from build123d import *

# Parameters (mm, degrees)
SKETCH_1_R                = 7
EXTRUDE_1_DEPTH           = 54
SKETCH_2_R                = 5
EXTRUDE_2_DEPTH           = 7
CHAMFER_1_SIZE            = 1
SKETCH_3_R                = 10
EXTRUDE_3_DEPTH           = 2
SKETCH_4_R                = 6
EXTRUDE_4_DEPTH           = 25
SKETCH_7_R                = 10
EXTRUDE_5_DEPTH           = 4.3
SKETCH_9_R                = 10
SKETCH_9_R_2              = 6
CUT_EXTRUDE_3_DEPTH       = 1.3
SKETCH_11_R               = 27
SKETCH_11_R_2             = 10
EXTRUDE_6_DEPTH           = 5
SKETCH_12_R               = 9.5
SKETCH_12_R_2             = 6
EXTRUDE_7_DEPTH           = 30
SKETCH_14_R               = 2.5
CUT_EXTRUDE_4_DEPTH       = 10
CUT_EXTRUDE_5_DEPTH       = 30
CHAMFER_2_SIZE            = 1
HOLE_WIZARD_M3_1_D        = 2.5
HOLE_WIZARD_M3_1_DEPTH    = 18.5
HOLE_WIZARD_M3_1_TIP      = 0.751075774
SKETCH_22_W               = 38.47112098
SKETCH_22_H               = 24.703275639
CUT_EXTRUDE_10_DEPTH      = 28
CUT_EXTRUDE_10_DEPTH_BACK = 28
SKETCH_24_R               = 9.5
EXTRUDE_9_DEPTH           = 10.3
SKETCH_25_R               = 7.5
EXTRUDE_10_DEPTH          = 17
SKETCH_26_W               = 19.870375241
SKETCH_26_H               = 17.333591793
CUT_EXTRUDE_11_DEPTH      = 28
CUT_EXTRUDE_11_DEPTH_BACK = 28
SKETCH_27_R               = 9.5
EXTRUDE_11_DEPTH          = 7.7
SKETCH_29_R               = 7.5
EXTRUDE_12_DEPTH          = 10
CUT_EXTRUDE_12_REACH      = 82
HOLE_WIZARD_M4_1_D        = 3.3
CHAMFER_4_SIZE            = 1
SKETCH_33_R               = 9.5
SKETCH_33_R_2             = 8.5
CUT_EXTRUDE_13_DEPTH      = 10
SKETCH_34_R               = 9.5
SKETCH_34_R_2             = 8.5
CUT_EXTRUDE_14_DEPTH      = 7.7
SKETCH_35_W               = 0.25
SKETCH_35_H               = 0.5
SKETCH_36_W               = 0.25
SKETCH_36_H               = 0.5


with BuildPart() as part:
    # 草图1 → 凸台-拉伸1 (new body)
    with BuildSketch(Plane.XY):
        Circle(SKETCH_1_R)
    extrude(amount=EXTRUDE_1_DEPTH)

    # 草图2 → 凸台-拉伸2 (add)
    with BuildSketch(Plane.XY.offset(54)):
        Circle(SKETCH_2_R)
    extrude(amount=EXTRUDE_2_DEPTH)

    # 倒角1
    chamfer_1_edges = [part.edges().sort_by_distance(p)[0] for p in [
        (-5, 0, 61),
    ]]
    chamfer(chamfer_1_edges, length=CHAMFER_1_SIZE)

    # 草图3 → 凸台-拉伸3 (add)
    with BuildSketch(Plane.XY.offset(42)):
        Circle(SKETCH_3_R)
    extrude(amount=-EXTRUDE_3_DEPTH)

    # 草图4 → 凸台-拉伸4 (add)
    with BuildSketch(Plane(origin=(0, 0, 0), x_dir=(-1, 0, 0), z_dir=(0, 0, -1))):
        Circle(SKETCH_4_R)
    extrude(amount=EXTRUDE_4_DEPTH)

    # 草图7 → 凸台-拉伸5 (add)
    with BuildSketch(Plane.XY.offset(42)):
        Circle(SKETCH_7_R)
    extrude(amount=EXTRUDE_5_DEPTH)

    # 草图9 → 切除-拉伸3 (cut)
    with BuildSketch(Plane(origin=(0, 0, 40), x_dir=(-1, 0, 0), z_dir=(0, 0, -1))):
        Circle(SKETCH_9_R)
        Circle(SKETCH_9_R_2, mode=Mode.SUBTRACT)
    extrude(amount=-CUT_EXTRUDE_3_DEPTH, mode=Mode.SUBTRACT)

    # 草图11 → 凸台-拉伸6 (add)
    with BuildSketch(Plane.XY.offset(46.3)):
        Circle(SKETCH_11_R)
        Circle(SKETCH_11_R_2, mode=Mode.SUBTRACT)
    extrude(amount=-EXTRUDE_6_DEPTH)

    # 草图12 → 凸台-拉伸7 (add)
    with BuildSketch(Plane(origin=(0, 0, 41.3), x_dir=(-1, 0, 0), z_dir=(0, 0, -1))):
        Circle(SKETCH_12_R)
        Circle(SKETCH_12_R_2, mode=Mode.SUBTRACT)
    extrude(amount=EXTRUDE_7_DEPTH)

    # 草图14 → 切除-拉伸4 (cut)
    with BuildSketch(Plane.XY.offset(46.3)):
        with Locations((22.5, 0)):
            Circle(SKETCH_14_R)
        with Locations((11.25, -19.485571585)):
            Circle(SKETCH_14_R)
        with Locations((-11.25, -19.485571585)):
            Circle(SKETCH_14_R)
        with Locations((-22.5, 0)):
            Circle(SKETCH_14_R)
        with Locations((-11.25, 19.485571585)):
            Circle(SKETCH_14_R)
        with Locations((11.25, 19.485571585)):
            Circle(SKETCH_14_R)
    extrude(amount=-CUT_EXTRUDE_4_DEPTH, mode=Mode.SUBTRACT)

    # 草图13 → 切除-拉伸5 (cut)
    with BuildSketch(Plane(origin=(0, 0, -25), x_dir=(-1, 0, 0), z_dir=(0, 0, -1))):
        with BuildLine():
            Line((2.15, 2.092247595), (2.15, -2.092247595))
            ThreePointArc((2.15, -2.092247595), (0, -3), (-2.15, -2.092247595))
            Line((-2.15, -2.092247595), (-2.15, 2.092247595))
            ThreePointArc((-2.15, 2.092247595), (0, 3), (2.15, 2.092247595))
        make_face()
    extrude(amount=-CUT_EXTRUDE_5_DEPTH, mode=Mode.SUBTRACT)

    # 倒角2
    chamfer_2_edges = [part.edges().sort_by_distance(p)[0] for p in [
        (6, 0, -25),
    ]]
    chamfer(chamfer_2_edges, length=CHAMFER_2_SIZE)

    # M3 螺纹孔1
    with Locations(Plane(origin=(7.85, 0, -17), x_dir=(0, 0, 1), z_dir=(1, 0, 0))):
        with Locations((0, 0)):
            Hole(HOLE_WIZARD_M3_1_D / 2, depth=HOLE_WIZARD_M3_1_DEPTH)
            with Locations((0, 0, -(HOLE_WIZARD_M3_1_DEPTH + HOLE_WIZARD_M3_1_TIP / 2))):  # 118° drill point
                Cone(0, HOLE_WIZARD_M3_1_D / 2, HOLE_WIZARD_M3_1_TIP, mode=Mode.SUBTRACT)

    # 草图22 → 切除-拉伸10 (cut, two sides)
    with BuildSketch(Plane(origin=(0, 0, 0), x_dir=(0, 0, -1), z_dir=(1, 0, 0))) as cut_extrude_10_sk:
        with Locations((7.93556049, 2.744045787)):
            Rectangle(SKETCH_22_W, SKETCH_22_H)
    extrude(amount=CUT_EXTRUDE_10_DEPTH, mode=Mode.SUBTRACT)
    extrude(cut_extrude_10_sk.sketch, amount=-CUT_EXTRUDE_10_DEPTH_BACK, mode=Mode.SUBTRACT)

    # 草图24 → 凸台-拉伸9 (add)
    with BuildSketch(Plane(origin=(0, 0, 11.3), x_dir=(-1, 0, 0), z_dir=(0, 0, -1))):
        Circle(SKETCH_24_R)
    extrude(amount=EXTRUDE_9_DEPTH)

    # 草图25 → 凸台-拉伸10 (add)
    with BuildSketch(Plane(origin=(0, 0, 1), x_dir=(-1, 0, 0), z_dir=(0, 0, -1))):
        Circle(SKETCH_25_R)
    extrude(amount=EXTRUDE_10_DEPTH)

    # 草图26 → 切除-拉伸11 (cut, two sides)
    with BuildSketch(Plane(origin=(0, 0, 0), x_dir=(0, 0, -1), z_dir=(1, 0, 0))) as cut_extrude_11_sk:
        with Locations((-56.23518762, 1.256529054)):
            Rectangle(SKETCH_26_W, SKETCH_26_H)
    extrude(amount=CUT_EXTRUDE_11_DEPTH, mode=Mode.SUBTRACT)
    extrude(cut_extrude_11_sk.sketch, amount=-CUT_EXTRUDE_11_DEPTH_BACK, mode=Mode.SUBTRACT)

    # 草图27 → 凸台-拉伸11 (add)
    with BuildSketch(Plane.XY.offset(46.3)):
        Circle(SKETCH_27_R)
    extrude(amount=EXTRUDE_11_DEPTH)

    # 草图29 → 凸台-拉伸12 (add)
    with BuildSketch(Plane.XY.offset(54)):
        Circle(SKETCH_29_R)
    extrude(amount=EXTRUDE_12_DEPTH)

    # 草图30 → 切除-拉伸12 (cut, up to next)
    with BuildSketch(Plane(origin=(0, 0, -16), x_dir=(-1, 0, 0), z_dir=(0, 0, -1)), mode=Mode.PRIVATE) as cut_extrude_12_sk1:
        with BuildLine():
            Line((4.05, 2.932149382), (4.05, -2.932149382))
            ThreePointArc((4.05, -2.932149382), (-5, 0), (4.05, 2.932149382))
        make_face()
    cut_extrude_12_tool1 = extrude(cut_extrude_12_sk1.sketch, amount=-CUT_EXTRUDE_12_REACH, mode=Mode.PRIVATE) & part.part
    add(cut_extrude_12_tool1.solids().sort_by_distance((0.224834, 0, -16))[0], mode=Mode.SUBTRACT)

    # M4 螺纹孔1 (through all)
    with Locations(Plane.ZY.offset(9.5)):
        with Locations((-10, 0)):
            Hole(HOLE_WIZARD_M4_1_D / 2)

    # 倒角4
    chamfer_4_edges = [part.edges().sort_by_distance(p)[0] for p in [
        (7.5, 0, -16),
        (-7.5, 0, 64),
    ]]
    chamfer(chamfer_4_edges, length=CHAMFER_4_SIZE)

    # 草图33 → 切除-拉伸13 (cut)
    with BuildSketch(Plane(origin=(0, 0, 1), x_dir=(-1, 0, 0), z_dir=(0, 0, -1))):
        Circle(SKETCH_33_R)
        Circle(SKETCH_33_R_2, mode=Mode.SUBTRACT)
    extrude(amount=-CUT_EXTRUDE_13_DEPTH, mode=Mode.SUBTRACT)

    # 草图34 → 切除-拉伸14 (cut)
    with BuildSketch(Plane.XY.offset(54)):
        Circle(SKETCH_34_R)
        Circle(SKETCH_34_R_2, mode=Mode.SUBTRACT)
    extrude(amount=-CUT_EXTRUDE_14_DEPTH, mode=Mode.SUBTRACT)

    # 草图35 → 切除-旋转1 (revolve, cut)
    with BuildSketch(Plane(origin=(0, 0, 0), x_dir=(1, 0, 0), z_dir=(0, 1, 0))):
        with Locations((7.375, -0.75)):
            Rectangle(SKETCH_35_W, SKETCH_35_H)
    revolve(axis=Axis((0, 0, 1), (0, 0, -1)), mode=Mode.SUBTRACT)

    # 草图36 → 切除-旋转2 (revolve, cut)
    with BuildSketch(Plane(origin=(0, 0, 0), x_dir=(1, 0, 0), z_dir=(0, 1, 0))):
        with Locations((7.375, -54.25)):
            Rectangle(SKETCH_36_W, SKETCH_36_H)
    revolve(axis=Axis((0, 0, 54), (0, 0, 1)), mode=Mode.SUBTRACT)


solid = part.part
CAD build for the part. Positions are in the model's coordinates, mm. A direction names the side the tool comes from. Round coordinates to 2 decimals unless told otherwise and drop trailing zeros. Loops run counter-clockwise (first coordinate to the right, second up) from the corner with the lowest first, then second, coordinate; pieces in that order, holes last.
(1) Which spindle directions (+Z, -Z, +X, -X, +Y, -Y) get a long thin tool onto all of the face, cutting with end or side? Do faces 4 (the cylindrical face through (-25, 0, 44)), 5 (the cylindrical face through (-7.493, 0.33, 58.69)), 6 (the flat face through (-7, -3, 1)). Say none if no direction does.
(2) Cut at C-C (z = -10). Give the cut face in (x, y), plus the area to 3 significant figures.
(3) Drop flat-ended pins along their axis: pin 1 (6 mm diameter, centred on x = -11.25, y = -19.49, fed in from -Z); pin 2 (5 mm diameter, centred on x = -1.5, z = 16.5, fed in from -Y); pin 3 (8 mm diameter, centred on x = 11.25, y = -19.49, fed in from +Z); pin 4 (15 mm diameter, centred on x = 1, y = -3, fed in from -Z). Give the stop position or say it passes through.
(4) Wall check: line 1 along Y through (x, z) = (0, 40); line 2 along Y through (x, z) = (-11.25, 43.75); line 3 along Y through (x, z) = (11, 44). Give the ranges that are in metal, low to high.
(5) Cut at D-D (y = 0). State how many separate pieces and enclosed holes the cut face has, plus the area to 3 significant figures.
(6) Cut at B-B (x = 11.25). Give the cut face in (y, z), plus the area to 3 significant figures.
(7) Two-plate mould, pull along X, no slides. Class faces 1 (the cylindrical face through (-11.575, -17.007, 43.835)), 2 (the cylindrical face through (-5.751, -0.632, -11.524)), 3 (the cylindrical face through (4.57, 7.167, 50.204)): +X half, -X half, draft (parallel to the pull), parting line (faces both ways), or undercut.
(8) Cut at A-A (x = -22.5). Give the cut face in (y, z), plus the area to 3 significant figures.
Findings below:
1. face 4: +Z, -Z
1. face 5: +Z
1. face 6: none
2. outline: (-7.32, -1.65) arc R7.5 ccw to (7.32, -1.65) - (4.72, -1.65) arc R5 cw to (-4.05, -2.93) - (-4.05, -1.65) - close; (-7.32, 1.65) - (-4.05, 1.65) - (-4.05, 2.93) arc R5 cw to (4.72, 1.65) - (7.32, 1.65) arc R7.5 ccw to start
2. area: 82.4 mm2
3. pin 1: stops at z = 41.3
3. pin 2: stops at y = -9.5
3. pin 3: stops at z = 46.3
3. pin 4: stops at z = -16
4. line 1: y = -9.5 to -5, 5 to 9.5
4. line 2: y = -24.54 to -21.99, -16.99 to 16.99, 21.99 to 24.54
4. line 3: y = -24.66 to -21.97, -17 to 17, 21.97 to 24.66
5. separate pieces: 6
5. enclosed holes: 0
5. area: 755 mm2
6. outline: (-24.54, 41.3) - (-21.99, 41.3) - (-21.99, 46.3) - (-24.54, 46.3) - close; (-16.99, 41.3) - (16.99, 41.3) - (16.99, 46.3) - (-16.99, 46.3) - close; (21.99, 41.3) - (24.54, 41.3) - (24.54, 46.3) - (21.99, 46.3) - close
6. area: 195 mm2
7. face 1: undercut
7. face 2: draft
7. face 3: parting line
8. outline: (-14.92, 41.3) - (-2.5, 41.3) - (-2.5, 46.3) - (-14.92, 46.3) - close; (2.5, 41.3) - (14.92, 41.3) - (14.92, 46.3) - (2.5, 46.3) - close
8. area: 124 mm2
